from build123d import *

# Parameters (mm, degrees)
SKETCH1_W           = 790.575
SKETCH1_H           = 608.0125
BOSS_EXTRUDE1_DEPTH = 19.05
SKETCH2_W           = 88.9
SKETCH2_H           = 38.1
SKETCH2_W_2         = 141.2875
CUT_EXTRUDE1_DEPTH  = 20.05
CHAMFER1_SIZE       = 2.54


with BuildPart() as part:
    # Sketch1 → Boss-Extrude1 (new body)
    with BuildSketch(Plane(origin=(0, 0, 0), x_dir=(1, 0, 0), z_dir=(0, 1, 0))):
        with Locations((395.2875, 304.00625)):
            Rectangle(SKETCH1_W, SKETCH1_H)
    extrude(amount=BOSS_EXTRUDE1_DEPTH)

    # Sketch2 → Cut-Extrude1 (cut, through all)
    with BuildSketch(Plane(origin=(0, 19.05, 0), x_dir=(1, 0, 0), z_dir=(0, 1, 0))):
        with Locations((693.7375, 588.9625)):
            Rectangle(SKETCH2_W, SKETCH2_H)
        with Locations((70.64375, 588.9625)):
            Rectangle(SKETCH2_W_2, SKETCH2_H)
        with Locations((70.64375, 19.05)):
            Rectangle(SKETCH2_W_2, SKETCH2_H)
        with Locations((693.7375, 19.05)):
            Rectangle(SKETCH2_W, SKETCH2_H)
    extrude(amount=-CUT_EXTRUDE1_DEPTH, mode=Mode.SUBTRACT)

    # Chamfer1
    chamfer1_edges = [part.edges().sort_by_distance(p)[0] for p in [
        (790.575, 19.05, -304.00625),
        (764.38125, 19.05, -608.0125),
        (0, 19.05, -304.00625),
        (395.2875, 19.05, 0),
        (764.38125, 19.05, 0),
        (395.2875, 19.05, -608.0125),
        (693.7375, 19.05, -38.1),
        (649.2875, 19.05, -19.05),
        (738.1875, 19.05, -19.05),
        (141.2875, 19.05, -19.05),
        (70.64375, 19.05, -38.1),
        (70.64375, 19.05, -569.9125),
        (141.2875, 19.05, -588.9625),
        (738.1875, 19.05, -588.9625),
        (649.2875, 19.05, -588.9625),
        (693.7375, 19.05, -569.9125),
    ]]
    chamfer(chamfer1_edges, length=CHAMFER1_SIZE)


solid = part.part
Check sheet for the modelled part. Datum: model origin and axes. Units: mm. A direction names the side the tool comes from. Round coordinates to 2 decimals unless told otherwise and drop trailing zeros. Loops run counter-clockwise (first coordinate to the right, second up) from the corner with the lowest first, then second, coordinate; pieces in that order, holes last. Notation, with made-up numbers: M -10,57.5 L 40,57.5 A18 ccw 40,65.5 Z; hole C -21.75,-19.5 d8. An arc over 180 degrees is marked long. One line per question, with ' | ' between items. Start each with the question number.
Item 1: Gauge pin test, flat ends, axial feed: pin 1 Ø5 at (x, y) = (82, 6) entering from +Z; pin 2 Ø5 at (y, z) = (6.5, -17.5) entering from -X. Record the tip position at first contact, or that the pin passes through.
Item 2: Section check B-B (x = 64.5). Record the boundary of the cut face in (y, z), and give its area (3 significant figures).
Item 3: Scan lines: probe 1 along Z at (x, y) = (122.5, 11); probe 2 along Z at (x, y) = (673, 17); probe 3 along X at (y, z) = (17, -182) (3 decimals). Record each from-to range of solid material in increasing order.
Item 4: Section check A-A (y = 7.5). Record the boundary of the cut face in (x, z) (1 decimal).
Item 5: Set-up check for faces 5 (the face through (649.287, 8, -19)), 6 (the face through (70, 8, -38.1)), 7 (the face through (738.188, 8, -589)), 8 (the face through (70, 8, -569.912)): record each of +Z, -Z, +X, -X, +Y, -Y from which the full face is reachable in a straight line by a thin tool's end or side.
Item 6: Release check for a two-part mould opening along X. For faces 1 (the face through (0, 8, -300)), 2 (the face through (764, 8, 0)), 3 (the face through (649.287, 8, -589)), 4 (the face through (790.575, 8, -300)) record: released by +X, released by -X, zero draft, split by the parting line, or undercut.
Worked out:
1) pin 1: z = -38.1 | pin 2: x = 141.29
2) outline: M 0,-569.91 L 16.51,-569.91 L 19.05,-567.37 L 19.05,-40.64 L 16.51,-38.1 L 0,-38.1 Z | area: 10,100 mm^2
3) probe 1: -569.91 to -38.1 | probe 2: -569.42 to -38.59 | probe 3: 0.49 to 790.085
4) outline: M 0,-569.9 L 141.3,-569.9 L 141.3,-608 L 649.3,-608 L 649.3,-569.9 L 738.2,-569.9 L 738.2,-608 L 790.6,-608 L 790.6,0 L 738.2,0 L 738.2,-38.1 L 649.3,-38.1 L 649.3,0 L 141.3,0 L 141.3,-38.1 L 0,-38.1 Z
5) face 5: +Z, +Y, -Y | face 6: +Z, -X, +Y, -Y | face 7: -Z, +Y, -Y | face 8: -Z, -X, +Y, -Y
6) face 1: released by -X | face 2: zero draft | face 3: undercut | face 4: released by +X
